Check sheet for the modelled part. Datum: model origin and axes. Units: mm. A direction names the side the tool comes from. Coordinates: 2 decimals unless noted, no trailing zeros. Loops run counter-clockwise (first coordinate to the right, second up) from the corner with the lowest first, then second, coordinate; pieces in that order, holes last. Notation, with made-up numbers: M 70,-19 L 97,-19 A17 cw 97,-8 Z; hole C 20,-9.75 d5. An arc over 180 degrees is marked long. Answer in a Markdown table with one row per item. Add a question column.
```python
from build123d import *

# Parameters (mm, degrees)
F1_DEPTH = 10
F2_DEPTH = 2.5


with BuildPart() as f1:
    # F0 (on Front) → F1 (new body)
    with BuildSketch(Plane.XZ):
        Polygon((-88.664238, 0), (0, 0), (0, 10), (-14.142136, 10), (-88.664238, 10), align=None)
        Polygon((-14.142136, 10), (0, 10), (-68.013943, 78.013943), (-75.085011, 70.942875), align=None)
    extrude(amount=F1_DEPTH)

    # F0 (on Front) → F2 (join)
    with BuildSketch(Plane.XZ):
        Polygon((-68.013943, 78.013943), (0, 10), (3.535534, 13.535534), (-64.478409, 81.549477), align=None)
    extrude(amount=F2_DEPTH)


solid = f1.part
```
Q1. Cross-section at C-C (z = 20.5). Record the cut outline in (x, y).
Q2. Thickness scan on L1, parallel to Y at x = -49.5, z = 66; L2, parallel to Z at x = -64, y = -7.25; L3, parallel to Z at x = -51.5, y = -8. Record the ranges inside material, lowest first.
Q3. Access from +Z, -Z, +X, -X, +Y, -Y to the whole of each face (thin tool, end or side, straight path). Record for faces 1 (the face through (-51, -5, 10)), 2 (the face through (-30, -1.23, 47.07)), 3 (the face through (-34, -6, 44)), 4 (the face through (0, -5, 5)).
Q4. Cross-section at B-B (y = -1.5). Record the cut outline in (x, z), plus the area to 3 significant figures.
Q5. Mould release check, pull along Z, two halves, no side actions. Record for faces 5 (the face through (-45.04, -4.93, 40.9)), 6 (the face through (-45, -5, 0)), 7 (the face through (-32.5, 0, 28.9)): released by +Z, released by -Z, zero draft, split by the parting line, or undercut.
Q6. Cross-section at A-A (x = -20.5). Record the cut outline in (y, z), plus the area to 3 significant figures.
Q7. Cross-section at D-D (z = 74). Record the cut outline in (x, y).
Q8. Go/stop test with flat-tipped pins: pin 1 (5 mm diameter, centred on x = -45, y = -2, fed in from +Z); pin 2 (1 mm diameter, centred on y = -4.5, z = 24.5, fed in from -X); pin 3 (3 mm diameter, centred on y = -7, z = 4, fed in from +X). Record where each tip stops, or that it passes through.
Answer key:
| question | item | result |
|---|---|---|
| 1 | outline | M -24.64,-10 L -10.5,-10 L -10.5,-2.5 L -3.43,-2.5 L -3.43,0 L -24.64,0 Z |
| 2 | L1 | -2.5 to 0 |
| 2 | L2 | 0 to 10, 59.86 to 74 |
| 2 | L3 | 0 to 10, 47.36 to 61.5 |
| 3 | face 1 | -X, +Y, -Y |
| 3 | face 2 | +Z, +X, +Y, -Y |
| 3 | face 3 | +Z, +X, -Y |
| 3 | face 4 | -Z, +X, +Y, -Y |
| 4 | outline | M -88.66,0 L 0,0 L 0,10 L 3.54,13.54 L -64.48,81.55 L -75.09,70.94 L -14.14,10 L -88.66,10 Z |
| 4 | area | 2,280 mm^2 |
| 5 | face 5 | undercut |
| 5 | face 6 | released by -Z |
| 5 | face 7 | zero draft |
| 6 | outline | M -10,0 L 0,0 L 0,10 L -10,10 Z; M -10,16.36 L 0,16.36 L 0,37.57 L -2.5,37.57 L -2.5,30.5 L -10,30.5 Z |
| 6 | area | 259 mm^2 |
| 7 | outline | M -72.03,-10 L -64,-10 L -64,-2.5 L -56.93,-2.5 L -56.93,0 L -72.03,0 Z |
| 8 | pin 1 | z = 64.57 |
| 8 | pin 2 | x = -29.14 |
| 8 | pin 3 | x = 0 |
